Model file for the job. Use its own axes, mm. A direction names the side the tool comes from. Coordinates: 2 decimals unless noted, no trailing zeros. Write each loop counter-clockwise with the first axis right and the second up, starting at its lowest first coordinate (ties: lowest second). Pieces come first, ordered by that corner, then holes. Notation, with made-up numbers: (-24.75, 86.5) - (-17.75, 86.5) arc R24 ccw to (-17.75, 104.5) - close; hole circle Ø9 at (60.5, 5.5). An arc over 180 degrees is marked (long way). Put each result on its own line as item: value. Start each with the question number.
1. Drill centre lines: L1, parallel to Y at x = 0, z = -3.2; L2, parallel to Y at x = -36.25, z = -2.75; L3, parallel to X at y = -17.5, z = -1.7. Where is each one in solid material? Low to high. Write a range as from..to.
2. Saw through at B-B, the plane x = -36.25. Write the cut outline in (y, z), plus the area to 3 significant figures.
3. Drop flat-ended pins along their axis: P1, Ø0.9, axis at x = 0, y = 17, coming from the +Z side; P2, Ø3, axis at x = -11, y = 7, coming from the +Z side; P3, Ø6.5, axis at x = 36.25, y = -17.5, coming from the +Z side. Give the stop position or say it passes through.
4. Pull direction Y, two halves, no side cores. Call faces 1 (the face through (-0.27, -18.72, 1.97)), 2 (the face through (5, -10, 0)), 3 (the face through (10, 0, -8)), 4 (the face through (23.5, 0, -7)): released by +Y, released by -Y, zero draft, split by the parting line, or undercut.
5. Saw through at A-A, the plane x = -56. Write the cut outline in (y, z), plus the area to 3 significant figures.
6. Which spindle directions (+Z, -Z, +X, -X, +Y, -Y) get a long thin tool onto all of the face, cutting with end or side? Do faces 5 (the face through (75, 0, -6)), 6 (the face through (4, 0, -8)). Say none if no direction does.
```python
from build123d import *

# Parameters (mm, degrees)
F0_W      = 3
F0_H      = 1
F0_H_2    = 15
F1_DEPTH  = 10
F0_W_2    = 150.0000016391
F0_H_3    = 40.0000016391
F0_R      = 1.25
F0_R_2    = 2
F0_R_3    = 1.5
F0_R_4    = 1.75
F0_W_3    = 2.5
F0_H_4    = 7.5
F0_H_5    = 3
F0_H_6    = 10
F3_DEPTH  = 3
F5_DEPTH  = 7.6
F7_DEPTH  = 3
F8_DEPTH  = 4
F9_DEPTH  = 5
F10_W     = 150.0000016391
F10_H     = 40.0000016391
F10_W_2   = 73.2
F10_H_2   = 30
F10_W_3   = 2.6
F10_W_4   = 59.2
F11_DEPTH = 4
F13_R     = 2


with BuildPart() as f1:
    # F0 (on Top) → F1 (new body)
    with BuildSketch(Plane.XY):
        with Locations((-45, 8)):
            Rectangle(F0_W, F0_H)
        with Locations((-45, 0)):
            Rectangle(F0_W, F0_H_2)
        with Locations((-45, -8)):
            Rectangle(F0_W, F0_H)
    extrude(amount=-F1_DEPTH)

    # F2 (on face) → F3 (cut, through all)
    with BuildSketch(Plane(origin=(-46.5, 0, 0), x_dir=(0, -1, 0), z_dir=(-1, 0, 0))):
        with BuildLine():
            ThreePointArc((-7.3, 0), (0, -7.3), (7.3, 0))
            Line((7.3, 0), (-7.3, 0))
        make_face()
    extrude(amount=-F3_DEPTH, mode=Mode.SUBTRACT)


with BuildPart() as f1b:
    # F0 (on Top) → F1, piece 2 (new body)
    with BuildSketch(Plane.XY):
        Rectangle(F0_W_2, F0_H_3)
        with Locations((-72.5000004098, -17.5000004098)):
            Circle(F0_R, mode=Mode.SUBTRACT)
        with Locations((-36.2500004098, -17.5000004098)):
            Circle(F0_R_2, mode=Mode.SUBTRACT)
        with Locations((-4.098e-07, -17.5000004098)):
            Circle(F0_R, mode=Mode.SUBTRACT)
        with Locations((36.2499995902, -17.5000004098)):
            Circle(F0_R_2, mode=Mode.SUBTRACT)
        with Locations((72.4999995902, -17.5000004098)):
            Circle(F0_R, mode=Mode.SUBTRACT)
        Polygon((-70, -15), (-70, 15), (3.2, 15), (5.7, 15), (8.3, 15), (10.8, 15), (70, 15), (70, -15), (10.8, -15), (8.3, -15), (5.7, -15), (3.2, -15), align=None, mode=Mode.SUBTRACT)
        with Locations((-72.5000004098, 17.4999995902)):
            Circle(F0_R_3, mode=Mode.SUBTRACT)
        with Locations((-36.2500004098, 17.4999995902)):
            Circle(F0_R_4, mode=Mode.SUBTRACT)
        with Locations((-4.098e-07, 17.4999995902)):
            Circle(F0_R_3, mode=Mode.SUBTRACT)
        with Locations((36.2499995902, 17.4999995902)):
            Circle(F0_R_4, mode=Mode.SUBTRACT)
        with Locations((72.4999995902, 17.4999995902)):
            Circle(F0_R_3, mode=Mode.SUBTRACT)
        with Locations((9.55, 0)):
            Rectangle(F0_W_3, F0_H_2)
        with Locations((4.45, 0)):
            Rectangle(F0_W_3, F0_H_2)
        with Locations((4.45, 11.25)):
            Rectangle(F0_W_3, F0_H_4)
        with Locations((9.55, 11.25)):
            Rectangle(F0_W_3, F0_H_4)
        with Locations((4.45, -11.25)):
            Rectangle(F0_W_3, F0_H_4)
        with Locations((9.55, -11.25)):
            Rectangle(F0_W_3, F0_H_4)
        with Locations((-36.2500004098, -17.5000004098)):
            Circle(F0_R_2)
        with Locations((36.2499995902, -17.5000004098)):
            Circle(F0_R_2)
        with Locations((-36.2500004098, 17.4999995902)):
            Circle(F0_R_4)
        with Locations((36.2499995902, 17.4999995902)):
            Circle(F0_R_4)
        with Locations((72.4999995902, 17.4999995902)):
            Circle(F0_R_3)
        with Locations((-4.098e-07, 17.4999995902)):
            Circle(F0_R_3)
        with Locations((-72.5000004098, 17.4999995902)):
            Circle(F0_R_3)
        with Locations((-72.5000004098, -17.5000004098)):
            Circle(F0_R)
        with Locations((-4.098e-07, -17.5000004098)):
            Circle(F0_R)
        with Locations((72.4999995902, -17.5000004098)):
            Circle(F0_R)
    extrude(amount=-F1_DEPTH)

    # F4 (on face) → F5 (cut, through all)
    with BuildSketch(Plane(origin=(3.2, 0, 0), x_dir=(0, -1, 0), z_dir=(-1, 0, 0))):
        with BuildLine():
            ThreePointArc((-8, 0), (0, -8), (8, 0))
            Line((8, 0), (-8, 0))
        make_face()
    extrude(amount=-F5_DEPTH, mode=Mode.SUBTRACT)

    # F0 (on Top) → F8 (join)
    with BuildSketch(Plane.XY):
        with Locations((-72.5000004098, -17.5000004098)):
            Circle(F0_R)
        with Locations((-4.098e-07, -17.5000004098)):
            Circle(F0_R)
        with Locations((72.4999995902, -17.5000004098)):
            Circle(F0_R)
        with Locations((-36.2500004098, 17.4999995902)):
            Circle(F0_R_4)
        with Locations((36.2499995902, 17.4999995902)):
            Circle(F0_R_4)
    extrude(amount=F8_DEPTH)

    # F0 (on Top) → F9 (cut)
    with BuildSketch(Plane.XY):
        with Locations((-4.098e-07, 17.4999995902)):
            Circle(F0_R_3)
        with Locations((72.4999995902, 17.4999995902)):
            Circle(F0_R_3)
        with Locations((-72.5000004098, 17.4999995902)):
            Circle(F0_R_3)
        with Locations((-36.2500004098, -17.5000004098)):
            Circle(F0_R_2)
        with Locations((36.2499995902, -17.5000004098)):
            Circle(F0_R_2)
    extrude(amount=-F9_DEPTH, mode=Mode.SUBTRACT)


with BuildPart() as f1c:
    # F0 (on Top) → F1, piece 3 (new body)
    with BuildSketch(Plane.XY):
        with Locations((25, 6.5)):
            Rectangle(F0_W, F0_H_5)
        with Locations((25, 0)):
            Rectangle(F0_W, F0_H_6)
        with Locations((25, -6.5)):
            Rectangle(F0_W, F0_H_5)
    extrude(amount=-F1_DEPTH)

    # F6 (on face) → F7 (cut, through all)
    with BuildSketch(Plane(origin=(23.5, 0, 0), x_dir=(0, -1, 0), z_dir=(-1, 0, 0))):
        with BuildLine():
            ThreePointArc((-6, 0), (0, -6), (6, 0))
            Line((6, 0), (-6, 0))
        make_face()
    extrude(amount=-F7_DEPTH, mode=Mode.SUBTRACT)


with BuildPart() as f11:
    # F10 (on face) → F11 (new body)
    with BuildSketch(Plane(origin=(0, 0, -10), x_dir=(1, 0, 0), z_dir=(0, 0, -1))):
        Rectangle(F10_W, F10_H)
        with Locations((-33.4, 0)):
            Rectangle(F10_W_2, F10_H_2, mode=Mode.SUBTRACT)
        with Locations((7, 0)):
            Rectangle(F10_W_3, F10_H_2, mode=Mode.SUBTRACT)
        with Locations((40.4, 0)):
            Rectangle(F10_W_4, F10_H_2, mode=Mode.SUBTRACT)
        with Locations((-33.4, 0)):
            Rectangle(F10_W_2, F10_H_2)
        with Locations((40.4, 0)):
            Rectangle(F10_W_4, F10_H_2)
        with Locations((7, 0)):
            Rectangle(F10_W_3, F10_H_2)
    extrude(amount=F11_DEPTH)

    # F12: union F1c, F1b, F1
    add(f1c.part)
    add(f1b.part)
    add(f1.part)

    # F13
    f13_edges = [f11.edges().sort_by_distance(p)[0] for p in [
        (-75.000001, -20.000001, -7),
        (75.000001, -20.000001, -7),
        (75.000001, 20.000001, -7),
        (-75.000001, 20.000001, -7),
        (-75.000001, 0, -14),
        (0, -20.000001, -14),
        (0, 20.000001, -14),
        (75.000001, 0, -14),
    ]]
    fillet(f13_edges, radius=F13_R)


solid = f11.part
```
Final values:
1. L1: y = -20..-15, 15..16, 19..20
1. L2: y = -20..-19.5, -15.5..-15, 15..20
1. L3: x = -75..-38.25, -34.25..34.25, 38.25..75
2. outline: (-20, -12) arc R2 ccw to (-18, -14) - (18, -14) arc R2 ccw to (20, -12) - (20, 0) - (19.25, 0) - (19.25, 4) - (15.75, 4) - (15.75, 0) - (15, 0) - (15, -10) - (-15, -10) - (-15, 0) - (-15.5, 0) - (-15.5, -5) - (-19.5, -5) - (-19.5, 0) - (-20, 0) - close
2. area: 252 mm²
3. P1: stops at z = -5
3. P2: stops at z = -10
3. P3: stops at z = 0
4. face 1: split by the parting line
4. face 2: zero draft
4. face 3: undercut
4. face 4: undercut
5. outline: (-20, -12) arc R2 ccw to (-18, -14) - (18, -14) arc R2 ccw to (20, -12) - (20, 0) - (15, 0) - (15, -10) - (-15, -10) - (-15, 0) - (-20, 0) - close
5. area: 258 mm²
6. face 5: +Z, -Z, +X, +Y, -Y
6. face 6: +Z
